Autodesk Inventor part; units mm, degrees
ref_plane "YZ Plane" through (0, 0, 0) normal (1, 0, 0) x (0, 1, 0)
ref_plane "XZ Plane" through (0, 0, 0) normal (0, 1, 0) x (-1, 0, 0)
ref_plane "XY Plane" through (0, 0, 0) normal (0, 0, 1) x (1, 0, 0)
sketch "Sketch1" plane through (0, 0, 0) normal (0, 1, 0) x (-1, 0, 0)
  line L0 (0, 0) -> (0, -19.05)
  circle A0 centre (0, -19.05) radius 4
  circle A1 centre (0, 0) radius 25
  dimension "d0" = 19.05
  dimension "d1" = 8
  dimension "d2" = 50
extrude "Extrusion1" add sketch "Sketch1" along normal blind 5 contours A0 | A1
sketch "Sketch2" plane through (0, 5, 0) normal (0, 1, 0) x (1, 0, 0)
  line L0 (0, 0) -> (0, 19.05)
  circle A0 centre (0, 19.05) radius 3.9
  dimension "d5" = 19.05
  dimension "d6" = 7.8
extrude "Extrusion2" add sketch "Sketch2" along normal blind 9
sketch "Sketch4" plane through (0, 5, 0) normal (0, 1, 0) x (1, 0, 0)
  circle A0 centre (0, 0) radius 9.25
  dimension "d9" = 18.5
extrude "Extrusion3" cut sketch "Sketch4" against normal blind 2
sketch "Sketch5" plane through (0, 3, 0) normal (0, 1, 0) x (1, 0, 0)
  line L0 (0, 0) -> (0, -6)
  circle A0 centre (0, -6) radius 2.125
  dimension "d12" = 6
  dimension "d13" = 4.25
extrude "Extrusion4" cut sketch "Sketch5" against normal through all
pattern_circular "Circular Pattern1" count 4 over 360 about axis through (0, 0, 0) along (0, 1, 0) of "Extrusion4"
sketch "Sketch6" plane through (0, 0, 0) normal (0, -1, 0) x (1, 0, 0)
  circle A0 centre (0, 0) radius 9
  circle A1 centre (0, 0) radius 2.125
  dimension "d19" = 18
  dimension "d20" = 4.25
extrude "Extrusion5" cut sketch "Sketch6" against normal through all contours A1
sketch "Sketch7" plane through (0, 5, 0) normal (0, 1, 0) x (1, 0, 0)
  point P0 (0, 0)
sketch "Sketch8" plane through (0, 5, 0) normal (0, 1, 0) x (1, 0, 0)
  circle A0 centre (0, 0) radius 9.25
  circle A1 centre (0, 0) radius 25
extrude "Extrusion6" cut sketch "Sketch8" along normal through all both and the other way through all
properties part number "Picker"
Here's how the part is built. I have some questions about the finished solid (model axes, mm). Coordinates: 2 decimals unless noted, no trailing zeros. Order: outer loops, then holes, each group sorted by start corner. A loop starts at its lowest first (then second) coordinate and runs counter-clockwise, first axis right, second up. Notation, with made-up numbers: (69.5, 6.25) - (98.5, 6.25) arc R24 cw to (98.5, 19.25) - close; hole circle Ø11 at (24.25, 52.5). An arc over 180 degrees is marked (long way). One line per question, with ' | ' between items. Start each with the question number.
1. If we section it at A-A (x = 0): Write out the boundary of the cut face in (y, z) (3 decimals).
2. If we section it at C-C (y = 2.3): Write out the boundary of the cut face in (x, z) (3 decimals), and give its area (3 significant figures).
3. I'm going to push flat-ended pins straight in: pin 1 Ø1 at (y, z) = (2.5, 4) entering from +X; pin 2 Ø1 at (x, y) = (-5, 2.5) entering from +Z; pin 3 Ø1.5 at (x, y) = (3, 1.5) entering from -Z. Where does each tip first touch, or does it pass through?
4. Please list where these lines run through material, in increasing order: line 1 along Z through (x, y) = (0, 1.25) (3 decimals); line 2 along X through (y, z) = (2.8, 0.5); line 3 along Z through (x, y) = (1.5, 0.25). Write a range as [from, to].
5. If we section it at B-B (z = 0): Write out the boundary of the cut face in (x, y) (3 decimals).
6. If we mould it in two halves opening along Z, with no side actions, what happens to faces 1 (the cylindrical face through (-2.01, 1.52, 9.03)), 2 (the cylindrical face through (0.461, 1.521, -8.074)), 3 (the flat face through (-2, 0, -2))? For each: released by +Z, released by -Z, zero draft, split by the parting line, or undercut.
7. If we section it at D-D (x = 7): Write out the boundary of the cut face in (y, z) (3 decimals).
Model answer:
1) outline: (0, -9.25) - (3, -9.25) - (3, -8.125) - (0, -8.125) - close; (0, -3.875) - (3, -3.875) - (3, -2.125) - (0, -2.125) - close; (0, 2.125) - (3, 2.125) - (3, 3.875) - (0, 3.875) - close; (0, 8.125) - (3, 8.125) - (3, 9.25) - (0, 9.25) - close
2) outline: circle Ø18.5 at (0, 0); hole circle Ø4.25 at (-6, 0); hole circle Ø4.25 at (0, -6); hole circle Ø4.25 at (0, 0); hole circle Ø4.25 at (0, 6); hole circle Ø4.25 at (6, 0) | area: 198 mm²
3) pin 1: stops at x = 8.56 | pin 2: stops at z = 8.08 | pin 3: stops at z = -8.97
4) line 1: z = [-9.25, -8.125], [-3.875, -2.125], [2.125, 3.875], [8.125, 9.25] | line 2: x = [-9.24, -8.07], [-3.93, -2.07], [2.07, 3.93], [8.07, 9.24] | line 3: z = [-9.13, -7.51], [-4.49, -1.51], [1.51, 4.49], [7.51, 9.13]
5) outline: (-9.25, 0) - (-8.125, 0) - (-8.125, 3) - (-9.25, 3) - close; (-3.875, 0) - (-2.125, 0) - (-2.125, 3) - (-3.875, 3) - close; (2.125, 0) - (3.875, 0) - (3.875, 3) - (2.125, 3) - close; (8.125, 0) - (9.25, 0) - (9.25, 3) - (8.125, 3) - close
6) face 1: split by the parting line | face 2: undercut | face 3: zero draft
7) outline: (0, -6.047) - (3, -6.047) - (3, -1.875) - (0, -1.875) - close; (0, 1.875) - (3, 1.875) - (3, 6.047) - (0, 6.047) - close
